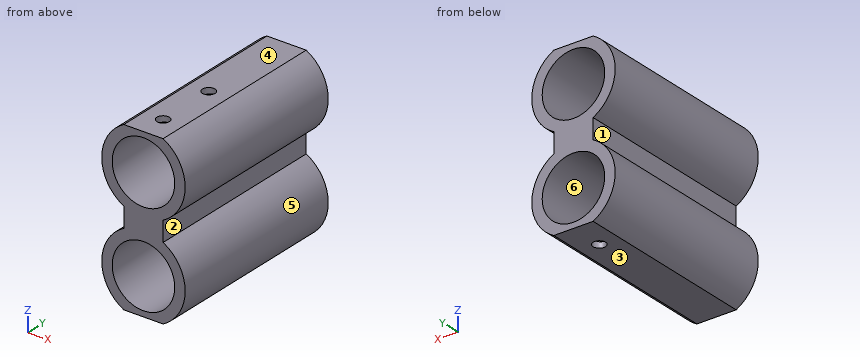
```python
from build123d import *

# Parameters (mm, degrees)
BOSS_EXTRUDE2_DEPTH = 45
SKETCH5_R           = 7.5
CUT_EXTRUDE2_DEPTH  = 48
SKETCH6_R           = 1.5
CUT_EXTRUDE3_DEPTH  = 5
SKETCH7_R           = 1.5
CUT_EXTRUDE4_DEPTH  = 10


with BuildPart() as part:
    # Sketch1 → Boss-Extrude2 (new body)
    with BuildSketch(Plane(origin=(0, 0, 0), x_dir=(1, 0, 0), z_dir=(0, 1, 0))):
        with BuildLine():
            Line((-4.710946187, 8.820826833), (4.710946187, 8.820826833))
            ThreePointArc((4.710946187, 8.820826833), (10, 0), (4.710946187, -8.820826833))
            Line((4.710946187, -8.820826833), (4.710946187, -13.627089834))
            ThreePointArc((4.710946187, -13.627089834), (10, -22.447916667), (4.710946187, -31.2687435))
            Line((4.710946187, -31.2687435), (-4.710946187, -31.2687435))
            ThreePointArc((-4.710946187, -31.2687435), (-10, -22.447916667), (-4.710946187, -13.627089834))
            Line((-4.710946187, -13.627089834), (-4.710946187, -8.820826833))
            ThreePointArc((-4.710946187, -8.820826833), (-10, 0), (-4.710946187, 8.820826833))
        make_face()
    extrude(amount=BOSS_EXTRUDE2_DEPTH)

    # Sketch5 → Cut-Extrude2 (cut)
    with BuildSketch(Plane(origin=(0, 45, 0), x_dir=(1, 0, 0), z_dir=(0, 1, 0))):
        Circle(SKETCH5_R)
        with Locations((0, -22.447916667)):
            Circle(SKETCH5_R)
    extrude(amount=-CUT_EXTRUDE2_DEPTH, mode=Mode.SUBTRACT)

    # Sketch6 → Cut-Extrude3 (cut)
    with BuildSketch(Plane.XY.offset(31.2687435)):
        with Locations((0, 20.532693815)):
            Circle(SKETCH6_R)
        with Locations((0, 6.178945615)):
            Circle(SKETCH6_R)
    extrude(amount=-CUT_EXTRUDE3_DEPTH, mode=Mode.SUBTRACT)

    # Sketch7 → Cut-Extrude4 (cut)
    with BuildSketch(Plane(origin=(0, 0, -8.820826833), x_dir=(-1, 0, 0), z_dir=(0, 0, -1))):
        with Locations((0, 36.852392065)):
            Circle(SKETCH7_R)
    extrude(amount=-CUT_EXTRUDE4_DEPTH, mode=Mode.SUBTRACT)


solid = part.part
```
Work out the finished part from the listing and answer in its coordinate system (mm). Face numbers are marked on the shaded views. A direction names the side the tool comes from. Give positions to 0.01 mm unless a question says otherwise; leave off trailing zeros. Order: outer loops, then holes, each group sorted by start corner. A loop starts at its lowest first (then second) coordinate and runs counter-clockwise, first axis right, second up.
1. Section B-B, the plane x = 0 is taken. Determine the outline of the cut face in (y, z).
Result sheet:
outline: (0, -8.82) - (35.35, -8.82) - (35.35, -7.5) - (0, -7.5) - close; (0, 7.5) - (45, 7.5) - (45, 14.95) - (0, 14.95) - close; (0, 29.95) - (4.68, 29.95) - (4.68, 31.27) - (0, 31.27) - close; (7.68, 29.95) - (19.03, 29.95) - (19.03, 31.27) - (7.68, 31.27) - close; (22.03, 29.95) - (45, 29.95) - (45, 31.27) - (22.03, 31.27) - close; (38.35, -8.82) - (45, -8.82) - (45, -7.5) - (38.35, -7.5) - close
2. Each of these flat-tipped pins is pushed along its axis until it touches: P1, Ø9, axis at x = 0, z = 22.45, coming from the -Y side; P2, Ø4, axis at x = 0, y = 20.53, coming from the +Z side; P3, Ø2.5, axis at y = 18.5, z = 10.5, coming from the -X side; P4, Ø1.4, axis at y = 33, z = 11, coming from the +X side. Where does it stop, or does it pass through?
Result sheet:
P1: passes through
P2: stops at z = 31.27
P3: stops at x = -4.71
P4: stops at x = 4.71
3. Section C-C, the plane x = 5.5 is taken. Determine the outline of the cut face in (y, z).
Result sheet:
outline: (0, -8.35) - (45, -8.35) - (45, -5.1) - (0, -5.1) - close; (0, 5.1) - (45, 5.1) - (45, 8.35) - (0, 8.35) - close; (0, 14.1) - (45, 14.1) - (45, 17.35) - (0, 17.35) - close; (0, 27.55) - (45, 27.55) - (45, 30.8) - (0, 30.8) - close
4. For the marked faces 1, 2 and 3, determine the directions among +Z, -Z, +X, -X, +Y, -Y from which every point of the face is accessible in a straight line to the end or side of a thin tool.
Result sheet:
face 1: -X, +Y, -Y
face 2: +X, +Y, -Y
face 3: -Z, +X, -X, +Y, -Y
5. Straight lines are drawn through the part: L1, parallel to Y at x = 0, z = 30.8; L2, parallel to Z at x = 0, y = 33; L3, parallel to Z at x = 0.25, y = 4. For each, find the intervals that lie inside material, in ascending order.
Result sheet:
L1: y = 0 to 4.68, 7.68 to 19.03, 22.03 to 45
L2: z = -8.82 to -7.5, 7.5 to 14.95, 29.95 to 31.27
L3: z = -8.82 to -7.5, 7.5 to 14.95, 29.94 to 31.27
6. Section A-A, the plane z = 0 is taken. Determine the outline of the cut face in (x, y).
Result sheet:
outline: (-10, 0) - (-7.5, 0) - (-7.5, 45) - (-10, 45) - close; (7.5, 0) - (10, 0) - (10, 45) - (7.5, 45) - close
7. Section D-D, the plane y = 40 is taken. Determine the outline of the cut face in (x, z).
Result sheet:
outline: (-4.71, -8.82) - (4.71, -8.82) arc R10 ccw to (4.71, 8.82) - (4.71, 13.63) arc R10 ccw to (4.71, 31.27) - (-4.71, 31.27) arc R10 ccw to (-4.71, 13.63) - (-4.71, 8.82) arc R10 ccw to start; hole circle Ø15 at (0, 0); hole circle Ø15 at (0, 22.45)
8. The mould has two halves that part along X. Classify the marked faces 4, 5 and 6: released by +X, released by -X, zero draft, split by the parting line, or undercut.
Result sheet:
face 4: zero draft
face 5: released by +X
face 6: undercut
